from build123d import *

# Parameters (mm, degrees)
F0_W     = 65
F0_H     = 50
F1_DEPTH = 10
F2_W     = 65
F2_H     = 20
F3_DEPTH = 35
F5_DEPTH = 5
F6_SIZE  = 10
F7_R     = 5
F8_DEPTH = 20.001


with BuildPart() as f1:
    # F0 (on Front) → F1 (new body)
    with BuildSketch(Plane.XZ):
        Rectangle(F0_W, F0_H)
    extrude(amount=F1_DEPTH)

    # F2 (on face) → F3 (join)
    with BuildSketch(Plane.XZ.offset(10)):
        with Locations((0, -15)):
            Rectangle(F2_W, F2_H)
    extrude(amount=F3_DEPTH)

    # F4 (on Right) → F5 (join, symmetric)
    with BuildSketch(Plane.YZ):
        Polygon((-45, -5), (-10, -5), (-10, 25), (-19.8282375932, 25), align=None)
    extrude(amount=F5_DEPTH, both=True)

    # F6
    f6_edges = [f1.edges().sort_by_distance(p)[0] for p in [
        (-32.5, -5, 25),
        (32.5, -5, 25),
    ]]
    chamfer(f6_edges, length=F6_SIZE)

    # F7 (on face) → F8 (cut, through all)
    with BuildSketch(Plane.XY.offset(-5)):
        with Locations((-18.5, -31)):
            Circle(F7_R)
        with Locations((18.5, -31)):
            Circle(F7_R)
    extrude(amount=-F8_DEPTH, mode=Mode.SUBTRACT)


solid = f1.part
The listing builds one solid part. Answer for the finished solid, in the listing's coordinates (mm). A direction names the side the tool comes from. Round coordinates to 2 decimals unless told otherwise and drop trailing zeros. Loops run counter-clockwise (first coordinate to the right, second up) from the corner with the lowest first, then second, coordinate; pieces in that order, holes last. Notation, with made-up numbers: M 64,26 L 113,26 A9 cw 113,38 Z; hole C -35.75,20.5 d4. An arc over 180 degrees is marked long. Write each question's results on one line, items separated by ' | '. Start each with the question number.
1) Straight lines are drawn through the part: probe 1 along Y at (x, z) = (-18.5, -15.75); probe 2 along X at (y, z) = (-33, -21.5); probe 3 along Z at (x, y) = (-19, -15). For each, find the intervals that lie inside material, in ascending order.
2) Determine the mould class of faces 1 (the flat face through (0, -45, -15)), 2 (the flat face through (19, -23, -5)), 3 (the cylindrical face through (17.42, -35.88, -14.86)), 4 (the cylindrical face through (-19.58, -35.88, -14.86)) for opening direction Y: pulls with the +Y half, pulls with the -Y half, needs draft (parallel to the pull), parting line crosses it, or undercut.
3) Find section D-D on x = 27.5. Write down the section's boundary in (y, z).
4) Find section A-A on x = -18.5. Write down the section's boundary in (y, z).
5) Which of the six approach directions +Z, -Z, +X, -X, +Y, -Y give full straight-line access (tool end or side, diameter ignored) to faces 5 (the flat face through (0, -22, -25)), 6 (the flat face through (-5, -24, 7)), 7 (the flat face through (19, -10, 10))?
6) Each of these flat-tipped pins is pushed along its axis until it touches: pin 1 (14 mm diameter, centred on x = -17.5, y = -19, fed in from +Z); pin 2 (8 mm diameter, centred on x = 7.5, z = 1, fed in from -Y); pin 3 (5 mm diameter, centred on x = -15.5, z = 5, fed in from +Y); pin 4 (8 mm diameter, centred on x = 12, z = 15.5, fed in from -Y). Where does it stop, or does it pass through?
7) Find section B-B on z = -9. Write down the section's boundary in (x, y), plus the area to 3 significant figures.
8) Find section C-C on y = -30. Write down the section's boundary in (x, z), plus the area to 3 significant figures.
Final values:
1) probe 1: -45 to -36, -26 to 0 | probe 2: -32.5 to -23.08, -13.92 to 13.92, 23.08 to 32.5 | probe 3: -25 to -5
2) face 1: pulls with the -Y half | face 2: needs draft | face 3: undercut | face 4: undercut
3) outline: M -45,-25 L 0,-25 L 0,20 L -10,20 L -10,-5 L -45,-5 Z
4) outline: M -45,-25 L -36,-25 L -36,-5 L -45,-5 Z; M -26,-25 L 0,-25 L 0,25 L -10,25 L -10,-5 L -26,-5 Z
5) face 5: -Z, +X, -X, +Y, -Y | face 6: +Z, -X, -Y | face 7: +Z, +X, -Y
6) pin 1: z = -5 | pin 2: y = -42.59 | pin 3: y = 0 | pin 4: y = -10
7) outline: M -32.5,-45 L 32.5,-45 L 32.5,0 L -32.5,0 Z; hole C -18.5,-31 d10; hole C 18.5,-31 d10 | area: 2,770 mm²
8) outline: M -32.5,-25 L -23.4,-25 L -23.4,-5 L -32.5,-5 Z; M -13.6,-25 L 13.6,-25 L 13.6,-5 L 5,-5 L 5,12.88 L -5,12.88 L -5,-5 L -13.6,-5 Z; M 23.4,-25 L 32.5,-25 L 32.5,-5 L 23.4,-5 Z | area: 1,090 mm²
